from build123d import *

# Parameters (mm, degrees)
SKETCH2_W            = 1900
SKETCH2_H            = 40
BASE_FLANGE1_DEPTH   = 8
EDGE_FLANGE1_START   = -950
EDGE_FLANGE1_DEPTH   = 1900
EDGE_FLANGE1_2_DEPTH = 1900


# Read off the part's stored shape, not the designer's step: Edge-Flange1
# Sheet-metal steps are written as plain solids
with BuildPart() as part:
    # Sketch2 → Base-Flange1 (new body)
    with BuildSketch(Plane(origin=(0, 0, 0), x_dir=(1, 0, 0), z_dir=(0, 1, 0))):
        with Locations((0, 20)):
            Rectangle(SKETCH2_W, SKETCH2_H)
    extrude(amount=-BASE_FLANGE1_DEPTH)

    # Edge-Flange1 outline → Edge-Flange1 (cut)
    with BuildSketch(Plane.YZ.offset(EDGE_FLANGE1_START)):
        with BuildLine():
            ThreePointArc((-8, -10.77542358), (-6.328529058, -4.946311673), (-1.822082615, -0.88868907))
            Line((-1.822082615, -0.88868907), (0, 0))
            Line((0, 0), (-8, 0))
            Line((-8, 0), (-8, -10.77542358))
        make_face()
    extrude(amount=EDGE_FLANGE1_DEPTH, mode=Mode.SUBTRACT)

    # Edge-Flange1 2 outline → Edge-Flange1 2 (add)
    with BuildSketch(Plane.YZ.offset(EDGE_FLANGE1_START)):
        with BuildLine():
            Line((35.142114222, 17.139954337), (0, 0))
            Line((0, 0), (0, -10.77542358))
            ThreePointArc((0, -10.77542358), (0.455855712, -9.185665787), (1.68488656, -8.079041441))
            Line((1.68488656, -8.079041441), (38.649083397, 9.949601967))
            Line((38.649083397, 9.949601967), (35.142114222, 17.139954337))
        make_face()
    extrude(amount=EDGE_FLANGE1_2_DEPTH)


solid = part.part
Geometry check sheet. Reference: the model listing, model coordinates, mm. A direction names the side the tool comes from. Round coordinates to 2 decimals unless told otherwise and drop trailing zeros. Write each loop counter-clockwise with the first axis right and the second up, starting at its lowest first coordinate (ties: lowest second). Pieces come first, ordered by that corner, then holes.
Item 1: Section check B-B (z = -29.5). Record the boundary of the cut face in (x, y), plus the area to 3 significant figures.
Determined:
outline: (-950, -8) - (950, -8) - (950, 0) - (-950, 0) - close
area: 15,200 mm2
Item 2: Section check C-C (y = 17.5). Record the boundary of the cut face in (x, z), plus the area to 3 significant figures.
Determined:
outline: (-950, -0.37) - (950, -0.37) - (950, 8.54) - (-950, 8.54) - close
area: 16,900 mm2
Item 3: Material ranges on line 1 along Y through (x, z) = (-563.5, -36); line 2 along Y through (x, z) = (-811, -0.5); line 3 along Z through (x, y) = (-296, 30.5), recorded low to high.
Determined:
line 1: y = -8 to 0
line 2: y = -1.03 to 17.22
line 3: z = 5.98 to 14.88
Item 4: Access from +Z, -Z, +X, -X, +Y, -Y to the whole of each face (thin tool, end or side, straight path). Record for faces 1 (the face through (-13, 0, -26)), 2 (the face through (-13, -8, -26)).
Determined:
face 1: -Z, +X, -X, +Y
face 2: +Z, -Z, +X, -X, -Y
Item 5: Section check A-A (x = -694). Record the boundary of the cut face in (y, z).
Determined:
outline: (-8, -40) - (0, -40) - (0, -10.78) arc R3 cw to (1.68, -8.08) - (38.65, 9.95) - (35.14, 17.14) - (-1.82, -0.89) arc R11 ccw to (-8, -10.78) - close
Item 6: Go/stop test with flat-tipped pins: pin 1 Ø12 at (x, z) = (353.5, 0.5) entering from -Y; pin 2 Ø8 at (x, z) = (-219, 2.5) entering from -Y; pin 3 Ø2 at (x, z) = (-380, 8) entering from +Y. Record where each tip stops, or that it passes through.
Determined:
pin 1: stops at y = -6.65
pin 2: stops at y = -2.91
pin 3: stops at y = 36.7
